```python
from build123d import *

# Parameters (mm, degrees)
SKETCH1_R           = 7
BOSS_EXTRUDE1_DEPTH = 10
BOSS_EXTRUDE3_DEPTH = 5
CHAMFER2_SIZE       = 2
CHAMFER2_SIZE_2     = 3.464101615
SKETCH7_R           = 9.5
BOSS_EXTRUDE4_DEPTH = 3
CUT_EXTRUDE1_DEPTH  = 10
FILLET1_R           = 1


with BuildPart() as part:
    # Sketch1 → Boss-Extrude1 (new body)
    with BuildSketch(Plane(origin=(0, 0, 0), x_dir=(1, 0, 0), z_dir=(0, 1, 0))):
        with Locations(Location((0, 0, 0), (0, 0, 270))):
            Circle(SKETCH1_R)
    extrude(amount=BOSS_EXTRUDE1_DEPTH)

    # Sketch5 → Boss-Extrude3 (add)
    with BuildSketch(Plane(origin=(0, 10, 0), x_dir=(1, 0, 0), z_dir=(0, 1, 0))):
        with BuildLine():
            Line((-3.821979409, 3.955056687), (-5.161555406, 4.72846125))
            ThreePointArc((-5.161555406, 4.72846125), (-6.062177826, 3.5), (-6.675745266, 2.10580748))
            Line((-6.675745266, 2.10580748), (-5.336169269, 1.332402917))
            ThreePointArc((-5.336169269, 1.332402917), (-4.763139721, 2.75), (-3.821979409, 3.955056687))
        make_face()
        with BuildLine():
            Line((1.51418986, 5.287459604), (1.51418986, 6.83426873))
            ThreePointArc((1.51418986, 6.83426873), (0, 7), (-1.51418986, 6.83426873))
            Line((-1.51418986, 6.83426873), (-1.51418986, 5.287459604))
            ThreePointArc((-1.51418986, 5.287459604), (0, 5.5), (1.51418986, 5.287459604))
        make_face()
        with BuildLine():
            ThreePointArc((6.675745266, 2.10580748), (6.062177826, 3.5), (5.161555406, 4.72846125))
            Line((5.161555406, 4.72846125), (3.821979409, 3.955056687))
            ThreePointArc((3.821979409, 3.955056687), (4.763139721, 2.75), (5.336169269, 1.332402917))
            Line((5.336169269, 1.332402917), (6.675745266, 2.10580748))
        make_face()
        with BuildLine():
            ThreePointArc((5.161555406, -4.72846125), (6.062177826, -3.5), (6.675745266, -2.10580748))
            Line((6.675745266, -2.10580748), (5.336169269, -1.332402917))
            ThreePointArc((5.336169269, -1.332402917), (4.763139721, -2.75), (3.821979409, -3.955056687))
            Line((3.821979409, -3.955056687), (5.161555406, -4.72846125))
        make_face()
        with BuildLine():
            ThreePointArc((-1.51418986, -6.83426873), (0, -7), (1.51418986, -6.83426873))
            Line((1.51418986, -6.83426873), (1.51418986, -5.287459604))
            ThreePointArc((1.51418986, -5.287459604), (0, -5.5), (-1.51418986, -5.287459604))
            Line((-1.51418986, -5.287459604), (-1.51418986, -6.83426873))
        make_face()
        with BuildLine():
            Line((-5.336169269, -1.332402917), (-6.675745266, -2.10580748))
            ThreePointArc((-6.675745266, -2.10580748), (-6.062177826, -3.5), (-5.161555406, -4.72846125))
            Line((-5.161555406, -4.72846125), (-3.821979409, -3.955056687))
            ThreePointArc((-3.821979409, -3.955056687), (-4.763139721, -2.75), (-5.336169269, -1.332402917))
        make_face()
    extrude(amount=BOSS_EXTRUDE3_DEPTH)

    # Chamfer2
    # the kernel refuses this chamfer: 3.464101615, 2 mm, written as the material it takes off along each edge
    with BuildSketch(Plane(origin=(-1.51418986, 15, -15.796196671), x_dir=(-0.05789386240267136, -0.9983227437537926, 0), z_dir=(0, 0, 1)), Plane(origin=(12.92281267, 15, -9.20942522), x_dir=(-0.02894693120133557, -0.9983227437537926, -0.05013755556391421), z_dir=(-0.8660254037844396, 0, 0.4999999999999985)), Plane(origin=(14.43700253, 15, 6.58677145), x_dir=(0.02894693120133555, -0.9983227437537926, -0.05013755556391386), z_dir=(-0.8660254037844383, 0, -0.5000000000000009)), Plane(origin=(1.51418986, 15, 15.796196671), x_dir=(0.05789386240267136, -0.9983227437537926, 0), z_dir=(0, 0, -1)), Plane(origin=(-12.92281267, 15, 9.20942522), x_dir=(0.028946931201335627, -0.9983227437537926, 0.05013755556391417), z_dir=(0.866025403784439, 0, -0.4999999999999995)), Plane(origin=(-14.43700253, 15, -6.58677145), x_dir=(-0.028946931201335666, -0.9983227437537926, 0.05013755556391416), z_dir=(0.8660254037844386, 0, 0.5000000000000002))) as chamfer2_piece_1:
        Polygon((CHAMFER2_SIZE * 0.998322743754, CHAMFER2_SIZE * 0.0578938624027), (-CHAMFER2_SIZE_2 * 0.057893862405, CHAMFER2_SIZE_2 * 0.998322743793), (0, 0), align=None)
    extrude(amount=19.470665008, mode=Mode.SUBTRACT)

    # Sketch7 → Boss-Extrude4 (add)
    with BuildSketch(Plane.XZ):
        with Locations(Location((0, 0, 0), (0, 0, 270))):
            Circle(SKETCH7_R)
    extrude(amount=BOSS_EXTRUDE4_DEPTH)

    # Sketch6 → Cut-Extrude1 (cut)
    with BuildSketch(Plane.XZ.offset(3)):
        with BuildLine():
            Line((1.224744871, 1.25), (-1.224744871, 1.25))
            ThreePointArc((-1.224744871, 1.25), (0, -1.75), (1.224744871, 1.25))
        make_face()
    extrude(amount=-CUT_EXTRUDE1_DEPTH, mode=Mode.SUBTRACT)

    # Fillet1
    fillet1_edges = [part.edges().sort_by_distance(p)[0] for p in [
        (0, 0, -7),
    ]]
    fillet(fillet1_edges, radius=FILLET1_R)


solid = part.part
```
Design review of the part built by this model. Coordinates are the model's own, in mm. A direction names the side the tool comes from. Round coordinates to 2 decimals unless told otherwise and drop trailing zeros. Write each loop counter-clockwise with the first axis right and the second up, starting at its lowest first coordinate (ties: lowest second). Pieces come first, ordered by that corner, then holes.
Item 1: For faces 4 (the flat face through (-5.32, 13.86, 3.1)), 5 (the flat face through (4.501, 11.479, -4.347)), 6 (the flat face through (-1.514, 12, 6)), 7 (the cylindrical face through (4.774, 11.813, 2.731)), 8 (the flat face through (5.997, 12.341, -1.714)), list the 3-axis set-ups (+Z, -Z, +X, -X, +Y, -Y) from which the entire face can be reached by the end or side of a thin tool; tool diameter is ignored.
Item 2: We need section A-A on y = 3. Write out the cut boundary in (x, z), and give its area (3 significant figures).
Item 3: We need section C-C on y = -1. Write out the cut boundary in (x, z), and give its area (3 significant figures).
Item 4: For probe 1 along X at (y, z) = (5, 0); probe 2 along Z at (x, y) = (0, 4); probe 3 along Y at (x, z) = (-0.25, -3), list the stretches that pass through material, from the lowest coordinate up.
Item 5: The part is to be moulded in two halves that separate along Z. For faces 1 (the flat face through (-4.501, 11.479, 4.347)), 2 (the cylindrical face through (0, 11.8, 5.5)), 3 (the flat face through (1.514, 12, -6)), say which applies: +Z half, -Z half, draft (parallel to the pull), parting line (faces both ways), or undercut.
Item 6: We need section B-B on x = 0. Write out the cut boundary in (y, z), and give its area (3 significant figures).
Item 7: Clearance check with flat-ended pins moving along their axes: pin 1 Ø0.8 at (y, z) = (11.5, -5.5) entering from -X; pin 2 Ø2.5 at (x, y) = (0.5, 4) entering from -Z; pin 3 Ø0.8 at (y, z) = (11, 6) entering from +X. State where each tip first meets the part, or that it passes through.
Returned:
1. face 4: +Z, +Y
1. face 5: -Z, +Y
1. face 6: +Z, -Z, -X, +Y
1. face 7: +Y
1. face 8: +X, +Y
2. outline: circle Ø14 at (0, 0); hole (-1.22, 1.25) arc R1.75 ccw (long way) to (1.22, 1.25) - close
2. area: 145 mm2
3. outline: circle Ø19 at (0, 0); hole (-1.22, 1.25) arc R1.75 ccw (long way) to (1.22, 1.25) - close
3. area: 275 mm2
4. probe 1: x = -7 to -1.75, 1.75 to 7
4. probe 2: z = -7 to -1.75, 1.25 to 7
4. probe 3: y = -3 to 10
5. face 1: +Z half
5. face 2: undercut
5. face 3: draft
6. outline: (-3, -9.5) - (0, -9.5) - (0, -8) arc R1 cw to (1, -7) - (13.87, -7) - (13.87, -5.5) - (10, -5.5) - (10, 5.5) - (13.87, 5.5) - (13.87, 7) - (1, 7) arc R1 cw to (0, 8) - (0, 9.5) - (-3, 9.5) - (-3, 1.25) - (7, 1.25) - (7, -1.75) - (-3, -1.75) - close
6. area: 179 mm2
7. pin 1: stops at x = -1.51
7. pin 2: stops at z = -7
7. pin 3: stops at x = 1.51
